Work out the finished part from the listing and answer in its coordinate system (mm). A direction names the side the tool comes from. Coordinates: 2 decimals unless noted, no trailing zeros. Answer as CSV lines item,"result". Start each with the question number.
(1) The mould has two halves that part along X. Classify faces 1 (the flat face through (0, -50.5, 6)), 2 (the flat face through (29, -45, 0)), 3 (the cylindrical face through (52.937, -16.671, 9.86)): released by +X, released by -X, zero draft, split by the parting line, or undercut.
(2) Flat-ended cylindrical pins translate along their axes: P1, Ø4, axis at x = -32.53, y = 32.53, coming from the -Z side; P2, Ø6, axis at x = 44.5, z = 9.5, coming from the +Y side; P3, Ø3, axis at x = -8, y = -27, coming from the +Z side; P4, Ø6, axis at x = 32.53, y = 32.53, coming from the -Z side. Find the tip coordinate at first contact, or state that the pin passes through.
(3) Find the intervals of material crossed by L1, parallel to Y at x = 0, z = 0.7; L2, parallel to Y at x = -3, z = 6; L3, parallel to Z at x = -41, y = 23.5, in increasing order. Write a range as [from, to].
(4) For faces 4 (the cylindrical face through (-28, 21, 12)), 5 (the cylindrical face through (29.11, 26.7, 0.99)), 6 (the cylindrical face through (30.03, -32.42, 14.33)), determine the directions among +Z, -Z, +X, -X, +Y, -Y from which every point of the face is accessible in a straight line to the end or side of a thin tool.
(5) A cutting plane is placed at A-A on x = 0. Count the separate pieces of the cut face and the enclosed holes in it, then the cut area to 3 significant figures.
Autodesk Inventor part; units mm, degrees
ref_plane "YZ Plane" through (0, 0, 0) normal (1, 0, 0) x (0, 1, 0)
ref_plane "XZ Plane" through (0, 0, 0) normal (0, 1, 0) x (-1, 0, 0)
ref_plane "XY Plane" through (0, 0, 0) normal (0, 0, 1) x (1, 0, 0)
sketch "Sketch1" plane through (0, 0, 0) normal (0, 0, 1) x (1, 0, 0)
  circle A0 centre (0, 0) radius 13
  circle A1 centre (0, 0) radius 55.5
  dimension "d0" = 26
  dimension "d1" = 111
extrude "Extrusion1" add sketch "Sketch1" along normal blind 5
sketch "Sketch2" plane through (0, 0, 5) normal (0, 0, 1) x (1, 0, 0)
  circle A0 centre (0, 0) radius 35
  circle A1 centre (0, 0) radius 55.5
  dimension "d4" = 70
extrude "Extrusion2" add sketch "Sketch2" along normal blind 15
sketch "Sketch3" plane through (0, 0, 0) normal (0, 0, -1) x (-1, 0, 0)
  circle A0 centre (0, 0) radius 39.5
  circle A1 centre (0, 0) radius 53
  dimension "d7" = 79
  dimension "d8" = 106
extrude "Extrusion3" cut sketch "Sketch3" against normal blind 4
chamfer "Chamfer1" distance 2 angle 15 1 edges at (39.5, 0, 4) measured on face at (-39.3895, -2.9518, 2.6667)
chamfer "Chamfer2" distance 2 angle 15 1 edges at (53, 0, 4) measured on face at (37.1782, -37.7728, 2.6667)
sketch "Sketch5" plane through (0, 0, 20) normal (0, 0, 1) x (1, 0, 0)
  circle A0 centre (-46, 0) radius 2.5
  circle A1 centre (-32.5269, -32.5269) radius 2.5
  circle A2 centre (0, -46) radius 2.5
  circle A3 centre (32.5269, -32.5269) radius 2.5
  circle A4 centre (46, 0) radius 2.5
  circle A5 centre (32.5269, 32.5269) radius 2.5
  circle A6 centre (0, 46) radius 2.5
  circle A7 centre (-32.5269, 32.5269) radius 2.5
  point P0 (0, 0)
  dimension "d17" = 5
  dimension "d18" = 46
  dimension "d21" = 360
extrude "Extrusion4" cut sketch "Sketch5" against normal through all
sketch "Sketch6" plane through (0, 0, 4) normal (0, 0, -1) x (-1, 0, 0)
  circle A0 centre (-46, 0) radius 2.5
  line L0 (-46, -5.1962) -> (-50.5, -2.5981)
  line L1 (-50.5, -2.5981) -> (-50.5, 2.5981)
  line L2 (-50.5, 2.5981) -> (-46, 5.1962)
  line L3 (-46, 5.1962) -> (-41.5, 2.5981)
  line L4 (-41.5, 2.5981) -> (-41.5, -2.5981)
  line L5 (-41.5, -2.5981) -> (-46, -5.1962)
  line L6 (-28.8527, -36.2011) -> (-33.8718, -37.546)
  line L7 (-33.8718, -37.546) -> (-37.546, -33.8718)
  line L8 (-37.546, -33.8718) -> (-36.2011, -28.8527)
  line L9 (-36.2011, -28.8527) -> (-31.182, -27.5078)
  line L10 (-31.182, -27.5078) -> (-27.5078, -31.182)
  line L11 (-27.5078, -31.182) -> (-28.8527, -36.2011)
  line L12 (5.1962, -46) -> (2.5981, -50.5)
  line L13 (2.5981, -50.5) -> (-2.5981, -50.5)
  line L14 (-2.5981, -50.5) -> (-5.1962, -46)
  line L15 (-5.1962, -46) -> (-2.5981, -41.5)
  line L16 (-2.5981, -41.5) -> (2.5981, -41.5)
  line L17 (2.5981, -41.5) -> (5.1962, -46)
  line L18 (36.2011, -28.8527) -> (37.546, -33.8718)
  line L19 (37.546, -33.8718) -> (33.8718, -37.546)
  line L20 (33.8718, -37.546) -> (28.8527, -36.2011)
  line L21 (28.8527, -36.2011) -> (27.5078, -31.182)
  line L22 (27.5078, -31.182) -> (31.182, -27.5078)
  line L23 (31.182, -27.5078) -> (36.2011, -28.8527)
  line L24 (46, 5.1962) -> (50.5, 2.5981)
  line L25 (50.5, 2.5981) -> (50.5, -2.5981)
  line L26 (50.5, -2.5981) -> (46, -5.1962)
  line L27 (46, -5.1962) -> (41.5, -2.5981)
  line L28 (41.5, -2.5981) -> (41.5, 2.5981)
  line L29 (41.5, 2.5981) -> (46, 5.1962)
  line L30 (28.8527, 36.2011) -> (33.8718, 37.546)
  line L31 (33.8718, 37.546) -> (37.546, 33.8718)
  line L32 (37.546, 33.8718) -> (36.2011, 28.8527)
  line L33 (36.2011, 28.8527) -> (31.182, 27.5078)
  line L34 (31.182, 27.5078) -> (27.5078, 31.182)
  line L35 (27.5078, 31.182) -> (28.8527, 36.2011)
  line L36 (-5.1962, 46) -> (-2.5981, 50.5)
  line L37 (-2.5981, 50.5) -> (2.5981, 50.5)
  line L38 (2.5981, 50.5) -> (5.1962, 46)
  line L39 (5.1962, 46) -> (2.5981, 41.5)
  line L40 (2.5981, 41.5) -> (-2.5981, 41.5)
  line L41 (-2.5981, 41.5) -> (-5.1962, 46)
  line L42 (-36.2011, 28.8527) -> (-37.546, 33.8718)
  line L43 (-37.546, 33.8718) -> (-33.8718, 37.546)
  line L44 (-33.8718, 37.546) -> (-28.8527, 36.2011)
  line L45 (-28.8527, 36.2011) -> (-27.5078, 31.182)
  line L46 (-27.5078, 31.182) -> (-31.182, 27.5078)
  line L47 (-31.182, 27.5078) -> (-36.2011, 28.8527)
  point P0 (0, 0)
  point P1 (-32.5269, -32.5269)
  point P2 (0, -46)
  point P3 (32.5269, -32.5269)
  point P4 (46, 0)
  point P5 (32.5269, 32.5269)
  point P6 (0, 46)
  point P7 (-32.5269, 32.5269)
  dimension "d25" = 9
  dimension "d28" = 360
extrude "Extrusion5" cut sketch "Sketch6" against normal blind 4.5 contours A0 | L0 L1 L2 L3 L4 L5 | L6 L7 L8 L9 L10 L11 | L12 L13 L14 L15 L16 L17 | L18 L19 L20 L21 L22 L23 | L24 L25 L26 L27 L28 L29 | L30 L31 L32 L33 L34 L35 | L36 L37 L38 L39 L40 L41 | L42 L43 L44 L45 L46 L47
properties part number "CS02" material "ABS Plastic"
Here are the results:
1,face 1,"undercut"
1,face 2,"zero draft"
1,face 3,"split by the parting line"
2,P1,"passes through"
2,P2,"stops at y = 36.85"
2,P3,"stops at z = 5"
2,P4,"stops at z = 8.5"
3,L1,"y = [-55.5, -53], [-39.5, -13], [13, 39.5], [53, 55.5]"
3,L2,"y = [-55.42, -49.8], [-42.2, -34.87], [34.87, 42.2], [49.8, 55.42]"
3,L3,"z = [4, 20]"
4,face 4,"+Z"
4,face 5,"-Z"
4,face 6,"+Z, -Z"
5,separate pieces,"4"
5,enclosed holes,"0"
5,area,"738 mm^2"
